Check sheet for the modelled part. Datum: model origin and axes. Units: mm. A direction names the side the tool comes from. Round coordinates to 2 decimals unless told otherwise and drop trailing zeros. Order: outer loops, then holes, each group sorted by start corner. A loop starts at its lowest first (then second) coordinate and runs counter-clockwise, first axis right, second up.
```python
from build123d import *

# Parameters (mm, degrees)
SKETCH1_R                      = 3.75
BOSS_EXTRUDE1_DEPTH            = 100
BOSS_EXTRUDE2_DEPTH            = 35
BOSS_EXTRUDE2_DEPTH_BACK       = 35
SKETCH2_R                      = 7.5
CUT_EXTRUDE1_REACH             = 53.113
SKETCH3_W                      = 3.85
SKETCH3_H                      = 3.85
CUT_EXTRUDE1_DIRECTION_2_REACH = 53.113


with BuildPart() as part:
    # Sketch1 → Boss-Extrude1 (new body)
    with BuildSketch(Plane.XY):
        Circle(SKETCH1_R)
    extrude(amount=BOSS_EXTRUDE1_DEPTH)

    # Sketch2 → Boss-Extrude2 (add, two sides: drawn at the far end of the back side and taken through both)
    with BuildSketch(Plane(origin=(0, 0, 50), x_dir=(-1, 0, 0), z_dir=(0, 0, -1)).offset(-BOSS_EXTRUDE2_DEPTH_BACK)):
        Circle(SKETCH2_R)
    extrude(amount=BOSS_EXTRUDE2_DEPTH + BOSS_EXTRUDE2_DEPTH_BACK)

    # Cut-Extrude1: up to this face of the body (flat: up to its plane)
    cut_extrude1_end = Plane(part.part.faces().sort_by_distance((7.287867966, 0, 85))[0])
    # Sketch3 → Cut-Extrude1 (cut, up to the picked face)
    with BuildSketch(Plane(origin=(0, 0, 50), x_dir=(-1, 0, 0), z_dir=(0, 0, -1)), mode=Mode.PRIVATE) as cut_extrude1_sk1:
        with Locations((0, 7.5)):
            Rectangle(SKETCH3_W, SKETCH3_H)
    cut_extrude1_tool1 = split(extrude(cut_extrude1_sk1.sketch, amount=-CUT_EXTRUDE1_REACH, mode=Mode.PRIVATE), bisect_by=cut_extrude1_end, keep=Keep.BOTH, mode=Mode.PRIVATE)
    add(cut_extrude1_tool1.solids().sort_by(Axis((0, 7.5, 50), (0, 0, 1)))[0], mode=Mode.SUBTRACT)

    # Cut-Extrude1 direction 2: up to this face of the body (flat: up to its plane)
    cut_extrude1_direction_2_end = Plane(part.part.faces().sort_by_distance((7.287867966, 0, 15))[0])
    # Sketch3 → Cut-Extrude1 direction 2 (cut, up to the picked face)
    with BuildSketch(Plane(origin=(0, 0, 50), x_dir=(-1, 0, 0), z_dir=(0, 0, -1)), mode=Mode.PRIVATE) as cut_extrude1_direction_2_sk1:
        with Locations((0, 7.5)):
            Rectangle(SKETCH3_W, SKETCH3_H)
    cut_extrude1_direction_2_tool1 = split(extrude(cut_extrude1_direction_2_sk1.sketch, amount=CUT_EXTRUDE1_DIRECTION_2_REACH, mode=Mode.PRIVATE), bisect_by=cut_extrude1_direction_2_end, keep=Keep.BOTH, mode=Mode.PRIVATE)
    add(cut_extrude1_direction_2_tool1.solids().sort_by(Axis((0, 7.5, 50), (0, 0, -1)))[0], mode=Mode.SUBTRACT)


solid = part.part
```
Item 1: Sectioned sample at A-A (y = 0). Record the cut outline in (x, z).
Answer:
outline: (-7.5, 15) - (-3.75, 15) - (-3.75, 0) - (3.75, 0) - (3.75, 15) - (7.5, 15) - (7.5, 85) - (3.75, 85) - (3.75, 100) - (-3.75, 100) - (-3.75, 85) - (-7.5, 85) - close
Item 2: Release check for a two-part mould opening along X. For faces 4 (the flat face through (1.925, 6, 50)), 5 (the cylindrical face through (0.303, -7.494, 50.49)), 6 (the flat face through (-3, -3, 85)) record: released by +X, released by -X, zero draft, split by the parting line, or undercut.
Answer:
face 4: undercut
face 5: split by the parting line
face 6: zero draft
Item 3: Sectioned sample at C-C (z = 6). Record the cut outline in (x, y).
Answer:
outline: circle Ø7.5 at (0, 0)
Item 4: Go/stop test with flat-tipped pins: P1, Ø1.3, axis at y = 6.5, z = 36, coming from the +X side; P2, Ø1.5, axis at y = -5.5, z = 52, coming from the +X side; P3, Ø2, axis at x = -3.5, z = 23.5, coming from the -Y side. Record where each tip stops, or that it passes through.
Answer:
P1: stops at x = 4.69
P2: stops at x = 5.8
P3: stops at y = -7.07
Item 5: Scan lines: line 1 along Z through (x, y) = (3.25, -3.75); line 2 along X through (y, z) = (6, 42.5) (3 decimals); line 3 along X through (y, z) = (-0.5, 67.5). Record each from-to range of solid material in increasing order.
Answer:
line 1: z = 15 to 85
line 2: x = -4.5 to -1.925, 1.925 to 4.5
line 3: x = -7.48 to 7.48
Item 6: Sectioned sample at B-B (x = 0). Record the cut outline in (y, z) (3 decimals), and give its area (3 significant figures).
Answer:
outline: (-7.5, 15) - (-3.75, 15) - (-3.75, 0) - (3.75, 0) - (3.75, 15) - (5.575, 15) - (5.575, 85) - (3.75, 85) - (3.75, 100) - (-3.75, 100) - (-3.75, 85) - (-7.5, 85) - close
area: 1,140 mm2
Item 7: Access from +Z, -Z, +X, -X, +Y, -Y to the whole of each face (thin tool, end or side, straight path). Record for faces 1 (the cylindrical face through (-3.746, 0.165, 92.395)), 2 (the flat face through (-3, -3, 15)), 3 (the flat face through (0, 5.575, 50)).
Answer:
face 1: +Z
face 2: -Z
face 3: +Z, -Z, +Y
Item 8: Sectioned sample at D-D (x = -6). Record the cut outline in (y, z), and give its area (3 significant figures).
Answer:
outline: (-4.5, 15) - (4.5, 15) - (4.5, 85) - (-4.5, 85) - close
area: 630 mm2
